Verification items for the finished model (mm, model axes). Round coordinates to 2 decimals unless told otherwise and drop trailing zeros. Loops run counter-clockwise (first coordinate to the right, second up) from the corner with the lowest first, then second, coordinate; pieces in that order, holes last. Notation, with made-up numbers: (44, -14.5) - (68, -14.5) arc R27 ccw to (68, 24.5) - close; hole circle Ø6 at (39.25, 32). An arc over 180 degrees is marked (long way). Use a Markdown table: item, result. Add a question column.
```python
from build123d import *

# Parameters (mm, degrees)
F1_DEPTH = 5
F2_R     = 5
F3_R     = 5


with BuildPart() as f1:
    # F0 (on Front) → F1 (new body)
    with BuildSketch(Plane.XZ):
        Polygon((40.09773, -95), (15, -20), (8.25, -20), (8.25, -62.5), (-8.25, -62.5), (-8.25, -20), (-15, -20), (-39.90227, -95), (-35.90227, -95), (-35.90227, -100), (-25.90227, -100), (-25.90227, -95), (-9.90227, -95), (-9.90227, -100), (10.09773, -100), (10.09773, -95), (26.09773, -95), (26.09773, -100), (36.09773, -100), (36.09773, -95), align=None)
        Polygon((8.25, -20), (15, -20), (15, 20), (-15, 20), (-15, -20), (-8.25, -20), (-8.25, -12.5), (-8.25, 12.5), (8.25, 12.5), (8.25, -12.5), align=None)
    extrude(amount=F1_DEPTH)

    # F2
    f2_edges = [f1.edges().sort_by_distance(p)[0] for p in [
        (-15, -2.5, 20),
    ]]
    fillet(f2_edges, radius=F2_R)

    # F3
    f3_edges = [f1.edges().sort_by_distance(p)[0] for p in [
        (15, -2.5, 20),
    ]]
    fillet(f3_edges, radius=F3_R)


solid = f1.part
```
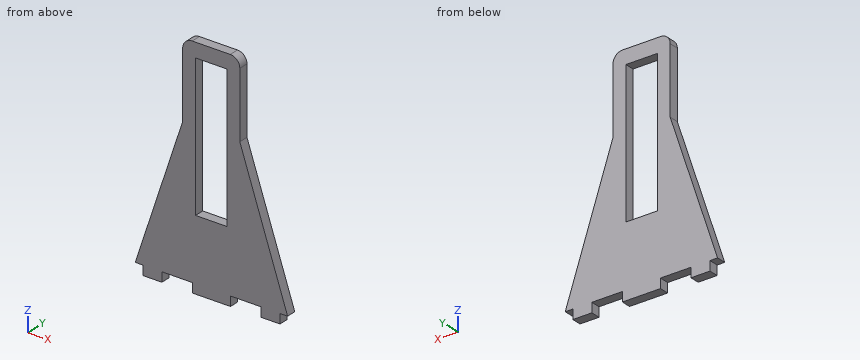
Q1. Thickness scan on line 1 along Z through (x, y) = (0.5, -1.75); line 2 along X through (y, z) = (-3.75, -5); line 3 along X through (y, z) = (-4.25, -24.5). Record the ranges inside material, lowest first.
Q2. Section check A-A on z = -11. Record the cut outline in (x, y).
Q3. Section check C-C on y = -3.3. Record the cut outline in (x, z), plus the area to 3 significant figures.
Q4. Go/stop test with flat-tipped pins: pin 1 Ø2.5 at (y, z) = (-1.5, -8.5) entering from -X; pin 2 Ø2 at (x, y) = (-38.5, -3) entering from -Z; pin 3 Ø1 at (y, z) = (-3, -68) entering from +X; pin 4 Ø10 at (x, z) = (3.5, -7) entering from +Y. Record where each tip stops, or that it passes through.
Q5. Section check B-B on x = -6.5. Record the cut outline in (y, z), plus the area to 3 significant figures.
Q6. Section check D-D on x = -23. Record the cut outline in (y, z).
Determined:
| question | item | result |
|---|---|---|
| 1 | line 1 | z = -100 to -62.5, 12.5 to 20 |
| 1 | line 2 | x = -15 to -8.25, 8.25 to 15 |
| 1 | line 3 | x = -16.49 to -8.25, 8.25 to 16.51 |
| 2 | outline | (-15, -5) - (-8.25, -5) - (-8.25, 0) - (-15, 0) - close; (8.25, -5) - (15, -5) - (15, 0) - (8.25, 0) - close |
| 3 | outline | (-39.9, -95) - (-35.9, -95) - (-35.9, -100) - (-25.9, -100) - (-25.9, -95) - (-9.9, -95) - (-9.9, -100) - (10.1, -100) - (10.1, -95) - (26.1, -95) - (26.1, -100) - (36.1, -100) - (36.1, -95) - (40.1, -95) - (15, -20) - (15, 15) arc R5 ccw to (10, 20) - (-10, 20) arc R5 ccw to (-15, 15) - (-15, -20) - close; hole (-8.25, -62.5) - (8.25, -62.5) - (8.25, 12.5) - (-8.25, 12.5) - close |
| 3 | area | 4,280 mm² |
| 4 | pin 1 | stops at x = -15 |
| 4 | pin 2 | stops at z = -95 |
| 4 | pin 3 | stops at x = 31.23 |
| 4 | pin 4 | stops at y = 0 |
| 5 | outline | (-5, -100) - (0, -100) - (0, -62.5) - (-5, -62.5) - close; (-5, 12.5) - (0, 12.5) - (0, 20) - (-5, 20) - close |
| 5 | area | 225 mm² |
| 6 | outline | (-5, -95) - (0, -95) - (0, -44.09) - (-5, -44.09) - close |
